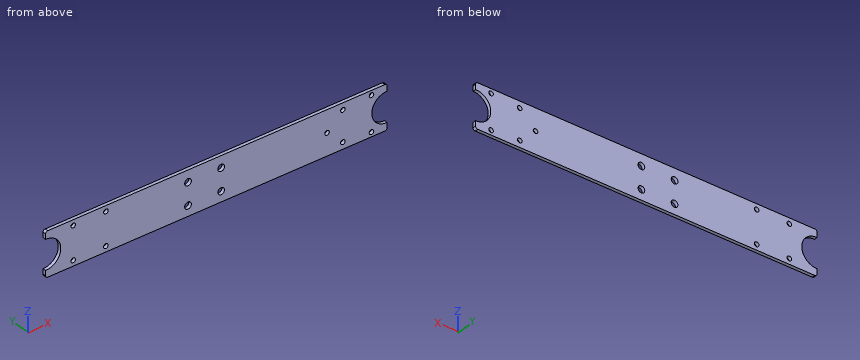
Autodesk Inventor part; units mm, degrees
ref_plane "YZ Plane" through (0, 0, 0) normal (1, 0, 0) x (0, 1, 0)
ref_plane "XZ Plane" through (0, 0, 0) normal (0, 1, 0) x (-1, 0, 0)
ref_plane "XY Plane" through (0, 0, 0) normal (0, 0, 1) x (1, 0, 0)
sketch "Sketch1" plane through (0, 0, 0) normal (0, 1, 0) x (-1, 0, 0)
  line L0 (-40.8289, 0) -> (-40.8289, -20.14)
  line L1 (-0.4496, -20.14) -> (-0.4496, 0)
  circle A0 centre (45.43, -2.545) radius 1.05
  circle A1 centre (45.43, -17.595) radius 1.05
  circle A2 centre (30.33, -2.545) radius 1.05
  circle A3 centre (30.33, -17.595) radius 1.05
  circle A4 centre (-22.8893, -5.31) radius 1.55
  circle A5 centre (-22.8893, -15.45) radius 1.55
  circle A6 centre (-7.5893, -5.31) radius 1.55
  circle A7 centre (-7.5893, -15.45) radius 1.55
  circle A8 centre (-92.3086, -18.07) radius 1.05
  circle A9 centre (-92.3086, -2.07) radius 1.05
  circle A10 centre (-79.0886, -17.07) radius 1.05
  circle A11 centre (-79.0886, -3.07) radius 1.05
  circle A12 centre (-71.7886, -10.07) radius 1.05
  arc A13 (58.19, -3.325) -> (58.19, -16.815) centre (57.93, -10.07) ccw
  line L2 (58.19, -16.815) -> (58.19, -19.14)
  arc A14 (-99.4686, -16.815) -> (-99.4686, -3.325) centre (-99.2086, -10.07) ccw
  line L3 (-99.4686, -19.14) -> (-99.4686, -16.815)
  arc A15 (-99.4686, -19.14) -> (-98.4686, -20.14) centre (-98.4686, -19.14) ccw
  line L4 (57.19, -20.14) -> (-98.4686, -20.14)
  arc A16 (57.19, -20.14) -> (58.19, -19.14) centre (57.19, -19.14) ccw
  line L5 (58.19, -1) -> (58.19, -3.325)
  arc A17 (58.19, -1) -> (57.19, 0) centre (57.19, -1) ccw
  line L6 (-98.4686, 0) -> (57.19, 0)
  arc A18 (-98.4686, 0) -> (-99.4686, -1) centre (-98.4686, -1) ccw
  line L7 (-99.4686, -3.325) -> (-99.4686, -1)
  line L8 (-41.2786, -20.14) -> (-41.2786, 0)
  line L9 (-40.3793, 0) -> (-40.3793, -20.14)
  line L10 (-0.8993, -20.14) -> (-0.8993, 0)
  line L11 (0, 0) -> (0, -20.14)
extrude "Extrusion1" add sketch "Sketch1" against normal blind 1.5
properties part number "axis_21_top_frame"
Work out the finished part from the listing and answer in its coordinate system (mm). Coordinates: 2 decimals unless noted, no trailing zeros.
1. A flat-ended cylindrical pin translates along its axis: pin 1 (1.3 mm diameter, centred on x = -45.43, z = -2.545, fed in from +Y). Find the tip coordinate at first contact, or state that the pin passes through.
Results list:
pin 1: passes through
2. Consider line 1 along X through (y, z) = (-0.8, -15.25); line 2 along X through (y, z) = (-0.5, -17.5); line 3 along X through (y, z) = (-0.45, -2.75). Determine where each line is inside the solid, lowest interval first.
Results list:
line 1: x = -53.6 to 6.05, 9.13 to 21.35, 24.43 to 94.88
line 2: x = -58.19 to -46.48, -44.38 to -31.38, -29.28 to 78.13, 80.05 to 91.43, 93.19 to 99.47
line 3: x = -58.19 to -46.46, -44.4 to -31.36, -29.3 to 78.09, 80.09 to 91.51, 93.11 to 99.47
3. The part is cut by section A-A, the plane y = -1.1. State how many separate pieces and enclosed holes the cut face has, and give its area (3 significant figures).
Results list:
separate pieces: 1
enclosed holes: 13
area: 2,960 mm2
